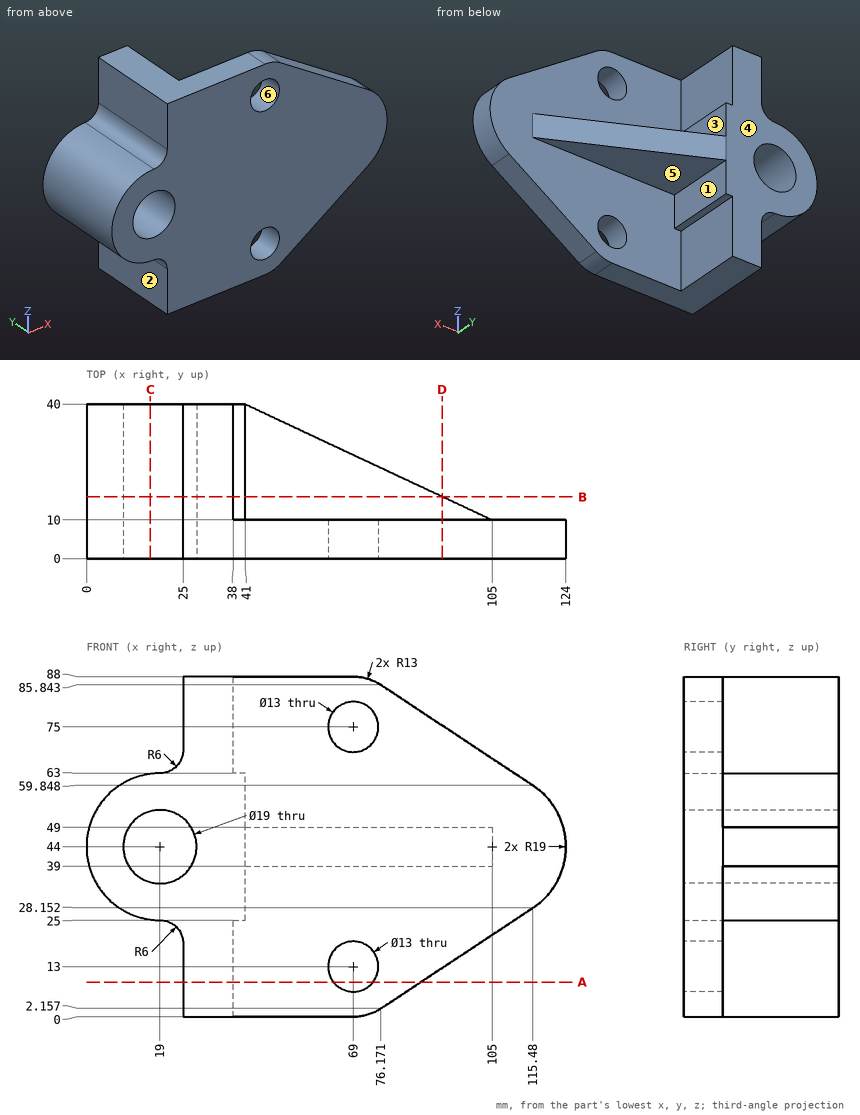
Here's the drawing with two shaded views (mm, measured from the low corner). I have some questions. A direction names the side the tool comes from. Round coordinates to 2 decimals unless told otherwise and drop trailing zeros. Write each loop counter-clockwise with the first axis right and the second up, starting at its lowest first coordinate (ties: lowest second). Pieces come first, ordered by that corner, then holes.
(1) Suppose I cut it at D-D on x = 92. Write out the boundary of the cut face in (y, z) (1 decimal).
Findings below:
outline: (0, 12.6) - (10, 12.6) - (10, 39) - (16.1, 39) - (16.1, 49) - (10, 49) - (10, 75.4) - (0, 75.4) - close
(2) Suppose I cut it at B-B on y = 16. Write out the boundary of the cut face in (x, z), and give its area (3 significant figures).
Findings below:
outline: (19, 25) arc R6 cw to (25, 19) - (25, 0) - (38, 0) - (38, 25) - (41, 25) - (41, 39) - (92.2, 39) - (92.2, 49) - (41, 49) - (41, 63) - (38, 63) - (38, 88) - (25, 88) - (25, 69) arc R6 cw to (19, 63) arc R19 ccw to start; hole circle Ø19 at (19, 44)
area: 2,300 mm2
(3) For pin 1 (8 mm diameter, centred on x = 69, z = 75, fed in from +Y); pin 2 (11 mm diameter, centred on y = 26, z = 55, fed in from +X); pin 3 (5 mm diameter, centred on y = 11, z = 70, fed in from -X); pin 4 (8 mm diameter, centred on y = 13, z = 35, fed in from +X) (1 decimal), each with a flat end and sliding along its axis, tell me the tip position at first contact or that it passes through.
Findings below:
pin 1: passes through
pin 2: stops at x = 41
pin 3: stops at x = 24.81
pin 4: stops at x = 122.9
(4) Suppose I cut it at A-A on z = 9. Write out the boundary of the cut face in (x, y), and give its area (3 significant figures).
Findings below:
outline: (25, 0) - (63.88, 0) - (63.88, 10) - (38, 10) - (38, 40) - (25, 40) - close; (74.12, 0) - (86.52, 0) - (86.52, 10) - (74.12, 10) - close
area: 903 mm2
(5) Which directions (+Z, -Z, +X, -X, +Y, -Y) give clear straight access to the entire face, cutting with the end or side of a thin tool? Please do the marked faces 1, 2 and 3.
Findings below:
face 1: -Z, +X, +Y
face 2: -Z, -X, +Y, -Y
face 3: +Z, +X, +Y
(6) Suppose I cut it at C-C on x = 16.5. Write out the boundary of the cut face in (y, z) (1 decimal).
Findings below:
outline: (0, 25.2) - (40, 25.2) - (40, 34.8) - (0, 34.8) - close; (0, 53.2) - (40, 53.2) - (40, 62.8) - (0, 62.8) - close
(7) If I drill on probe 1 along Z at (x, y) = (69, 2.25); probe 2 along Z at (x, y) = (19, 16); probe 3 along Y at (x, z) = (89, 25.5), over which ranges is the centre line in solid material (lowest first)?
Findings below:
probe 1: z = 0 to 6.5, 19.5 to 68.5, 81.5 to 88
probe 2: z = 25 to 34.5, 53.5 to 63
probe 3: y = 0 to 10
(8) Thinking about a two-plate mould opening in Z: for the marked faces 4, 5 and 6, which applies, +Z half, -Z half, draft (parallel to the pull), parting line (faces both ways), or undercut?
Findings below:
face 4: draft
face 5: -Z half
face 6: undercut
